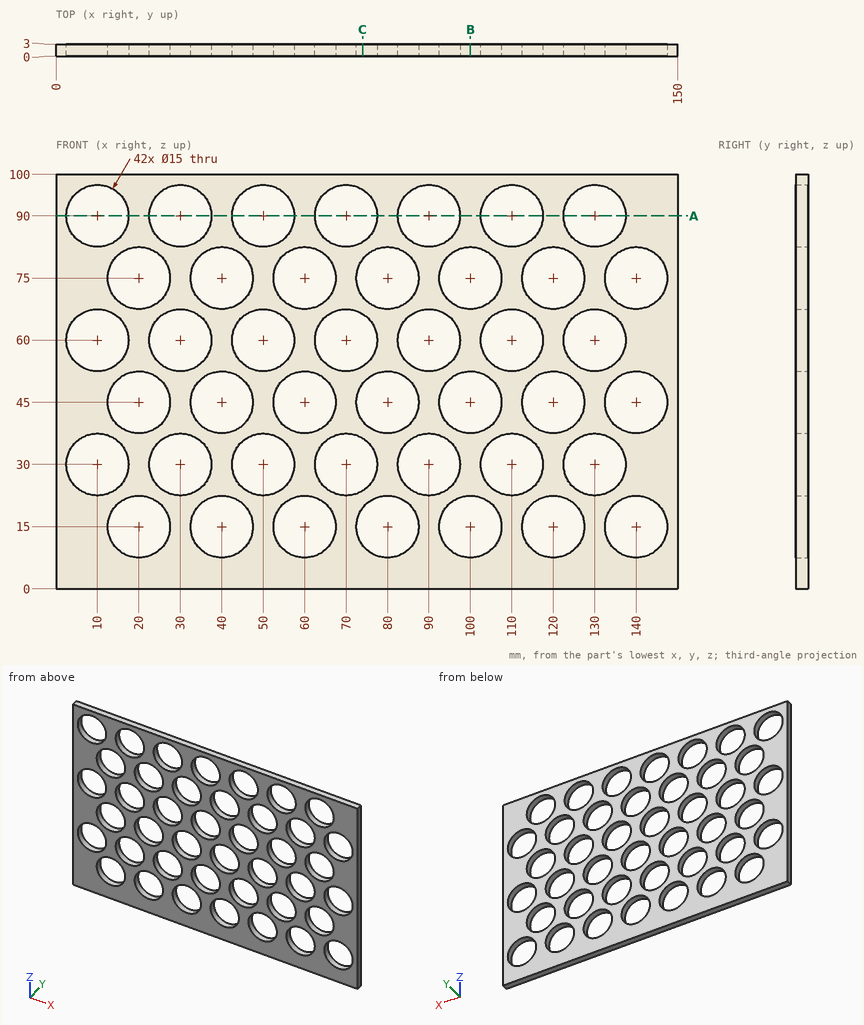
Input: dimensioned drawing with shaded views. Units: mm. Origin: part minimum x, y, z. Give positions to 0.01 mm unless a question says otherwise; leave off trailing zeros. Write each loop counter-clockwise with the first axis right and the second up, starting at its lowest first coordinate (ties: lowest second). Pieces come first, ordered by that corner, then holes.
1. Section query C-C, the plane x = 74. Return loops of the section in (y, z).
2. Pin query (flat end, axial travel): P1, Ø1, axis at x = 70, z = 68, coming from the -Y side. Return the tip coordinate at first contact, or that it passes through.
3. Line query: probe 1 along Z at (x, y) = (60, 1.3); probe 2 along Z at (x, y) = (50, 2.2). Output: solid intervals per line, ascending.
4. Section query A-A, the plane z = 90. Count the separate pieces of the cut face and the enclosed holes in it, then the cut area to 3 significant figures.
5. Section query B-B, the plane x = 100. Return loops of the section in (y, z), then the cut area to 3 significant figures.
Computed:
1. outline: (0, 0) - (3, 0) - (3, 10.5) - (0, 10.5) - close; (0, 19.5) - (3, 19.5) - (3, 23.66) - (0, 23.66) - close; (0, 36.34) - (3, 36.34) - (3, 40.5) - (0, 40.5) - close; (0, 49.5) - (3, 49.5) - (3, 53.66) - (0, 53.66) - close; (0, 66.34) - (3, 66.34) - (3, 70.5) - (0, 70.5) - close; (0, 79.5) - (3, 79.5) - (3, 83.66) - (0, 83.66) - close; (0, 96.34) - (3, 96.34) - (3, 100) - (0, 100) - close
2. P1: stops at y = 0
3. probe 1: z = 0 to 7.5, 22.5 to 37.5, 52.5 to 67.5, 82.5 to 100
3. probe 2: z = 0 to 22.5, 37.5 to 52.5, 67.5 to 82.5, 97.5 to 100
4. separate pieces: 8
4. enclosed holes: 0
4. area: 135 mm2
5. outline: (0, 0) - (3, 0) - (3, 7.5) - (0, 7.5) - close; (0, 22.5) - (3, 22.5) - (3, 37.5) - (0, 37.5) - close; (0, 52.5) - (3, 52.5) - (3, 67.5) - (0, 67.5) - close; (0, 82.5) - (3, 82.5) - (3, 100) - (0, 100) - close
5. area: 165 mm2
